from build123d import *

# Parameters (mm, degrees)
SKETCH1_W           = 9.525
SKETCH1_H           = 25.4
BOSS_EXTRUDE1_DEPTH = 25.4
SKETCH4_R           = 1.5875
CUT_EXTRUDE1_DEPTH  = 9.525


with BuildPart() as part:
    # Sketch1 → Boss-Extrude1 (new body)
    with BuildSketch(Plane(origin=(0, 0, 0), x_dir=(1, 0, 0), z_dir=(0, 1, 0))):
        with Locations((4.7625, 12.7)):
            Rectangle(SKETCH1_W, SKETCH1_H)
    extrude(amount=BOSS_EXTRUDE1_DEPTH)

    # Sketch4 → Cut-Extrude1 (cut)
    with BuildSketch(Plane.XZ):
        with Locations(Location((4.7625, -19.05, 0), (0, 0, 270))):
            Circle(SKETCH4_R)
        with Locations(Location((4.7625, -6.35, 0), (0, 0, 270))):
            Circle(SKETCH4_R)
    extrude(amount=-CUT_EXTRUDE1_DEPTH, mode=Mode.SUBTRACT)


solid = part.part
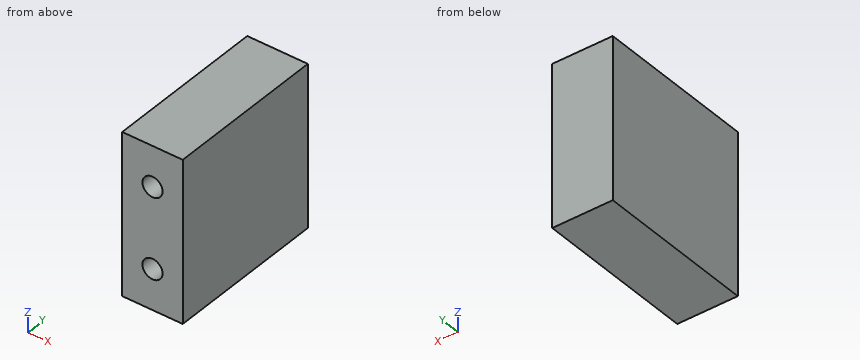
CAD build for the part. Positions are in the model's coordinates, mm. Coordinates: 2 decimals unless noted, no trailing zeros. Write each loop counter-clockwise with the first axis right and the second up, starting at its lowest first coordinate (ties: lowest second). Pieces come first, ordered by that corner, then holes. Notation, with made-up numbers: M 18,5 L 66,5 A18 cw 66,38 Z; hole C 4,52 d7. An arc over 180 degrees is marked long. Answer as a JSON object with one key per item and string values. Group by question number.
1) Saw through at A-A (z = -6.35). Write the cut outline in (x, y) (3 decimals), plus the area to 3 significant figures.
2) Saw through at C-C (z = -19). Write the cut outline in (x, y) (3 decimals), plus the area to 3 significant figures.
3) Wall check: line 1 (X direction, y = 6.5, z = -6.35) (3 decimals); line 2 (Z direction, x = 4.5, y = 4.5); line 3 (Y direction, x = 4.25, z = -5) (3 decimals). Give the ranges that are in metal, low to high. Write a range as from..to.
4) Pin check, flat tip, straight feed: pin 1 Ø4 at (x, z) = (4.76, -19.05) entering from -Y. Stop position of the tip, or through.
5) Saw through at B-B (y = 7.5). Give the number of separate pieces and of enclosed holes in the cut face, plus the area to 3 significant figures.
Values follow:
{
 "1": {"outline": "M 0,0 L 3.175,0 L 3.175,9.525 L 6.35,9.525 L 6.35,0 L 9.525,0 L 9.525,25.4 L 0,25.4 Z", "area": "212 mm2"},
 "2": {"outline": "M 0,0 L 3.176,0 L 3.176,9.525 L 6.349,9.525 L 6.349,0 L 9.525,0 L 9.525,25.4 L 0,25.4 Z", "area": "212 mm2"},
 "3": {"line 1": "x = 0..3.175, 6.35..9.525", "line 2": "z = -25.4..-20.62, -17.48..-7.92, -4.78..0", "line 3": "y = 9.525..25.4"},
 "4": {"pin 1": "stops at y = 0"},
 "5": {"separate pieces": "1", "enclosed holes": "2", "area": "226 mm2"}
}
